Build history of the part. All positions in model axes, mm. Round coordinates to 2 decimals unless told otherwise and drop trailing zeros. Write each loop counter-clockwise with the first axis right and the second up, starting at its lowest first coordinate (ties: lowest second). Pieces come first, ordered by that corner, then holes. Notation, with made-up numbers: M 76,28.5 L 121,28.5 A10 ccw 121,35.5 Z; hole C 63,60 d5. An arc over 180 degrees is marked long. Write item = value, one per line.
from build123d import *

# Parameters (mm, degrees)
SKETCH1_W             = 63.5
SKETCH1_H             = 38.1
BOSS_EXTRUDE1_DEPTH   = 6.35
SKETCH2_R             = 14.0462
SKETCH2_R_2           = 10.9474
CUT_EXTRUDE1_DEPTH    = 1.9558
F_8_CLEARANCE_HOLE1_D = 4.3053
FILLET1_R             = 0.127
FILLET2_R             = 0.254


with BuildPart() as part:
    # Sketch1 → Boss-Extrude1 (new body)
    with BuildSketch(Plane(origin=(0, 0, 0), x_dir=(1, 0, 0), z_dir=(0, 1, 0))):
        Rectangle(SKETCH1_W, SKETCH1_H)
    extrude(amount=BOSS_EXTRUDE1_DEPTH)

    # Sketch2 → Cut-Extrude1 (cut)
    with BuildSketch(Plane(origin=(0, 6.35, 0), x_dir=(1, 0, 0), z_dir=(0, 1, 0))):
        with Locations(Location((0, 0, 0), (0, 0, 270))):  # turned: the seam where the file's is
            Circle(SKETCH2_R)
        with Locations(Location((0, 0, 0), (0, 0, 270))):  # turned: the seam where the file's is
            Circle(SKETCH2_R_2, mode=Mode.SUBTRACT)
    extrude(amount=-CUT_EXTRUDE1_DEPTH, mode=Mode.SUBTRACT)

    # #8 Clearance Hole1 (through all)
    with Locations(Plane(origin=(0, 0, 0), x_dir=(-1, 0, 0), z_dir=(0, -1, 0))):
        with Locations((26.9875, -14.2875), (-26.9875, -14.2875), (-26.9875, 14.2875), (26.9875, 14.2875)):
            Hole(F_8_CLEARANCE_HOLE1_D / 2)

    # Fillet1
    fillet1_edges = [part.edges().sort_by_distance(p)[0] for p in [
        (0, 6.35, -14.0462),
        (0, 6.35, -10.9474),
    ]]
    fillet(fillet1_edges, radius=FILLET1_R)

    # Fillet2
    fillet2_edges = [part.edges().sort_by_distance(p)[0] for p in [
        (0, 4.3942, -14.0462),
        (0, 4.3942, -10.9474),
    ]]
    fillet(fillet2_edges, radius=FILLET2_R)


solid = part.part
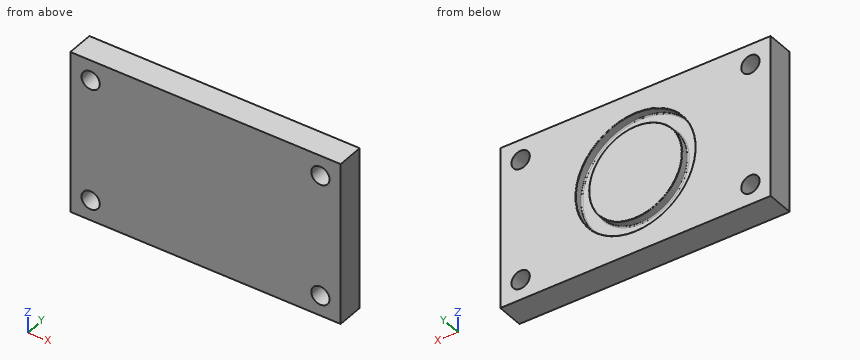
1. Band-saw the part on C-C (z = 0). List the corners of the cut face in (x, y), plus the area to 3 significant figures.
Responses:
outline = M -31.75,0 L 31.75,0 L 31.75,6.35 L 14.17,6.35 A0.13 ccw 14.05,6.22 L 14.05,4.65 A0.25 cw 13.79,4.39 L 11.2,4.39 A0.25 cw 10.95,4.65 L 10.95,6.22 A0.13 ccw 10.82,6.35 L -10.82,6.35 A0.13 ccw -10.95,6.22 L -10.95,4.65 A0.25 cw -11.2,4.39 L -13.79,4.39 A0.25 cw -14.05,4.65 L -14.05,6.22 A0.13 ccw -14.17,6.35 L -31.75,6.35 Z
area = 391 mm²
2. Band-saw the part on B-B (y = 5.5). List the corners of the cut face in (x, z).
Responses:
outline = M -31.75,-19.05 L 31.75,-19.05 L 31.75,19.05 L -31.75,19.05 Z; C 0,0 d21.89; hole C -26.99,-14.29 d4.31; hole C -26.99,14.29 d4.31; hole C 0,0 d28.09; hole C 26.99,-14.29 d4.31; hole C 26.99,14.29 d4.31
3. Band-saw the part on A-A (x = 0). List the corners of the cut face in (y, z), plus the area to 3 significant figures.
Responses:
outline = M 0,-19.05 L 6.35,-19.05 L 6.35,-14.17 A0.13 ccw 6.22,-14.05 L 4.65,-14.05 A0.25 cw 4.39,-13.79 L 4.39,-11.2 A0.25 cw 4.65,-10.95 L 6.22,-10.95 A0.13 ccw 6.35,-10.82 L 6.35,10.82 A0.13 ccw 6.22,10.95 L 4.65,10.95 A0.25 cw 4.39,11.2 L 4.39,13.79 A0.25 cw 4.65,14.05 L 6.22,14.05 A0.13 ccw 6.35,14.17 L 6.35,19.05 L 0,19.05 Z
area = 230 mm²
4. Band-saw the part on D-D (y = 2.5). List the corners of the cut face in (x, z).
Responses:
outline = M -31.75,-19.05 L 31.75,-19.05 L 31.75,19.05 L -31.75,19.05 Z; hole C -26.99,-14.29 d4.31; hole C -26.99,14.29 d4.31; hole C 26.99,-14.29 d4.31; hole C 26.99,14.29 d4.31
5. Probe probe 1 along Z at (x, y) = (-28, 1.75); probe 2 along Z at (x, y) = (4.5, 6); probe 3 along X at (y, z) = (5.5, -1). List the from-to ranges inside material, lowest first.
Responses:
probe_1 = -19.05 to -16.19, -12.39 to 12.39, 16.19 to 19.05
probe_2 = -19.05 to -13.31, -9.98 to 9.98, 13.31 to 19.05
probe_3 = -31.75 to -14.01, -10.9 to 10.9, 14.01 to 31.75
